Autodesk Inventor part; units mm, degrees
ref_plane "XZ Plane" through (0, 0, 0) normal (0, 1, 0) x (-1, 0, 0)
ref_plane "XY Plane" through (0, 0, 0) normal (0, 0, 1) x (1, 0, 0)
sketch "Эскиз1" plane through (0, 0, 0) normal (1, 0, 0) x (0, 1, 0)
  circle A0 centre (0, 0) radius 70
  circle A1 centre (0, 0) radius 82.5
  arc A2 (80.4212, 18.894) -> (80.3103, 18.8815) centre (82.3009, 1.7165) ccw
  circle A3 centre (0, 0) radius 97.5
  line L0 (142.5, 102) -> (108, 102)
  line L1 (0, -132.6) -> (0, 165.6)
  line L2 (142.5, 102) -> (142.5, 68)
  line L3 (108, 102) -> (108, 101.5)
  line L4 (108, 101.5) -> (0, 101.5)
  line L5 (-142.5, 102) -> (-108, 102)
  line L6 (-142.5, 102) -> (-142.5, 68)
  line L7 (-108, 102) -> (-108, 101.5)
  line L8 (-108, 101.5) -> (0, 101.5)
  arc A4 (11.7449, -38.2368) -> (27.2385, -29.2927) centre (0, 0) ccw
  arc A5 (-27.2416, -29.2898) -> (-11.749, -38.2356) centre (0, 0) ccw
  line L9 (-142.5, 68) -> (-69.8731, 68)
  line L10 (97.5, 0) -> (97.5, 68)
  line L11 (142.5, 68) -> (69.8731, 68)
  line L12 (-97.5, 0) -> (-97.5, 68)
  line L13 (117.5, 43) -> (117.5, 123)
  line L14 (-117.5, 43) -> (-117.5, 123)
  line L15 (133.5, 68) -> (117.5, 68)
  line L16 (117.5, 68) -> (117.5, 69)
  line L17 (117.5, 69) -> (133.5, 69)
  line L18 (133.5, 69) -> (133.5, 68)
  line L19 (128.5, 69) -> (117.5, 69)
  line L20 (117.5, 69) -> (117.5, 85)
  line L21 (128.5, 102) -> (128.5, 69)
  line L22 (133.5, 102) -> (117.5, 102)
  line L23 (117.5, 69) -> (101.5, 69)
  line L24 (101.5, 69) -> (101.5, 68)
  line L25 (106.5, 101.5) -> (106.5, 69)
  line L26 (-108, 102) -> (-108, 101.5)
  line L27 (-133.5, 68) -> (-117.5, 68)
  line L28 (-117.5, 68) -> (-117.5, 69)
  line L29 (-117.5, 69) -> (-133.5, 69)
  line L30 (-133.5, 69) -> (-133.5, 68)
  line L31 (-128.5, 69) -> (-117.5, 69)
  line L32 (-117.5, 69) -> (-117.5, 85)
  line L33 (-128.5, 102) -> (-128.5, 69)
  line L34 (-133.5, 102) -> (-117.5, 102)
  line L35 (-101.5, 69) -> (-101.5, 68)
  line L36 (-117.5, 69) -> (-101.5, 69)
  line L37 (-106.5, 101.5) -> (-106.5, 69)
  line L38 (117.5, 68) -> (117.5, 102)
  line L39 (-117.5, 68) -> (-117.5, 102)
  line L40 (0, 0) -> (69.6414, -69.6414)
  circle A6 centre (58.3363, -58.3363) radius 6.5
  circle A7 centre (58.3363, 58.3363) radius 6.5
  circle A8 centre (-58.3363, 58.3363) radius 6.5
  circle A9 centre (-58.3363, -58.3363) radius 6.5
  arc A10 (69.8731, 68) -> (-69.8731, 68) centre (0, 0) ccw
  line L41 (97.5, 68) -> (69.8731, 68)
  line L42 (-69.8731, 68) -> (-97.5, 68)
  line L43 (128.5, 69) -> (128.5, 102)
  line L44 (89, 68) -> (89, 101.5)
  arc A11 (83.0142, 68) -> (79.5188, 56.4182) centre (116.097, 51.6972) ccw
  arc A12 (79.5188, 56.4182) -> (62.6803, 74.6822) centre (0, 0) ccw
  line L45 (83.0142, 68) -> (83.0142, 84.568)
  line L46 (83.0142, 84.568) -> (89, 84.568)
  arc A13 (79.5188, 56.4182) -> (62.6803, 74.6822) centre (0, 0) ccw
  line L47 (-101.5, 69) -> (-101.5, 68)
  line L48 (-97.5, 68) -> (-69.8731, 68)
  arc A14 (-79.5188, 56.4182) -> (-83.0142, 68) centre (-116.097, 51.6972) ccw
  arc A15 (-62.6803, 74.6822) -> (-79.5188, 56.4182) centre (0, 0) ccw
  line L49 (-83.0142, 68) -> (-83.0142, 84.568)
  line L50 (-83.0142, 84.568) -> (-89, 84.568)
  arc A16 (-62.6803, 74.6822) -> (-79.5188, 56.4182) centre (0, 0) ccw
  line L51 (0, 97.5) -> (0, 101.5)
  line L52 (0, 101.5) -> (89, 101.5)
  line L53 (89, 101.5) -> (89, 84.568)
  arc A17 (62.6803, 74.6822) -> (0, 97.5) centre (0, 0) ccw
  arc A18 (89, 84.568) -> (47.9908, 67.1054) centre (89, 27.6838) ccw
  arc A19 (47.9908, 67.1054) -> (0, 82.5) centre (0, 0) ccw
  line L54 (79.5188, 56.4182) -> (60.3628, 70.1005)
  line L55 (60.3628, 70.1005) -> (47.9908, 67.1054)
  arc A20 (-47.9908, 67.1054) -> (-89, 84.568) centre (-89, 27.6838) ccw
  line L56 (-79.5188, 56.4182) -> (-59.1498, 66.8423)
  line L57 (-59.1498, 66.8423) -> (-47.9908, 67.1054)
  line L58 (0, 101.5) -> (-89, 101.5)
  line L59 (-89, 101.5) -> (-89, 84.568)
  arc A21 (-47.9908, 67.1054) -> (-89, 84.568) centre (-89, 27.6838) ccw
  arc A22 (0, 82.5) -> (-47.9908, 67.1054) centre (0, 0) ccw
  arc A23 (47.9908, 67.1054) -> (-47.9908, 67.1054) centre (0, 0) ccw
  point P0 (80.4117, 18.4447)
  point P1 (0, -97.5)
  point P2 (128.5, 85)
  point P3 (106.5, 85)
  point P4 (-128.5, 85)
  point P5 (-106.5, 85)
  point P6 (-89, 68)
  dimension "d0" = 140
  dimension "d4" = 165
  dimension "d19" = 195
  dimension "d20" = 199.5
  dimension "d22" = 285
  dimension "d23" = 216
  dimension "d24" = 0.5
  dimension "d46" = 34
  dimension "d64" = 235
  dimension "d65" = 16
  dimension "d66" = 11
  dimension "d67" = 1
  dimension "d70" = 45
  dimension "d71" = 13
  dimension "d74" = 360
  dimension "d84" = 12.5
extrude "Выдавливание1" add sketch "Эскиз1" along normal blind 34 and the other way blind 34 contours A0 L1 A1 A7 A6 L40 | A0 L1 A1 A9 A8 | L40 A6 A1 L1 A0 | A6 A1 L40 | L40 A1 A6 | A1 A9 | A1 A7 | A8 A1 picked at (57.6773, -55.9908) picked at (55.9908, -57.6773) picked at (-56.6588, -56.9353) picked at (56.9815, 56.6214) picked at (-56.6588, 56.9353)
extrude "Выдавливание2" add sketch "Эскиз1" along normal blind 34 and the other way blind 34 contours A0 L40 L1 | A0 L1 A1 A7 A6 L40 | L1 A0 | A0 L1 A1 A9 A8 | L40 A6 A1 L1 A0 | A0 L1 L40 | A6 A1 L40 | L40 A1 A6 | A1 A9 | A1 A7 | A8 A1 picked at (57.6773, -55.9908) picked at (55.9908, -57.6773) picked at (-56.6588, -56.9353) picked at (56.9815, 56.6214) picked at (-56.6588, 56.9353)
pattern_circular "Круговой массив1" count 6 over 360 about axis through (0, 0, 0) along (1, 0, 0) of "Выдавливание2"
extrude "Выдавливание3" add sketch "Эскиз1" along normal blind 33 and the other way blind 33 contours A0 L40 L1 | A0 L1 A1 A7 A6 L40 | L1 A0 | A0 L1 A1 A9 A8 | L40 A6 A1 L1 A0 | A0 L1 L40 | L1 A3 A18 A1 | A1 A20 A3 L1 | A6 A1 L40 | L40 A1 A6 | L1 A3 L56 L57 A1 A8 A9 | A1 A6 L40 A3 L1 | L55 L54 A3 L40 A6 A1 A7 | A18 A3 L54 L55 | L57 L56 A3 A20 | L40 A6 A1 | A1 A6 L40 | A9 A1 | A1 A9 | A7 A1 | A1 A7 | A8 A1 | A1 A8 | A11 L11 L10 A3 | A3 L11 A11
extrude "Выдавливание4" add sketch "Эскиз1" along normal blind 33 and the other way blind 33 contours L12 L9 A14 A3 | A14 L9 A3
extrude "Выдавливание7" add sketch "Эскиз1" along normal blind 33 and the other way blind 33 contours A0 L40 L1 | A0 L1 A1 A7 A6 L40 | L1 A0 | A0 L1 A1 A9 A8 | L40 A6 A1 L1 A0 | A0 L1 L40 | L1 A3 A18 A1 | A1 A20 A3 L1 | L1 A3 L56 L57 A1 A8 A9 | A1 A6 L40 A3 L1 | L55 L54 A3 L40 A6 A1 A7 | A18 A3 L54 L55 | L57 L56 A3 A20 | L1 L4 L44 L46 L45 A18 A3 | A3 A20 L49 L50 L59 L8 L1 | A18 L45 L11 A3 | A3 L9 L49 A20 | A18 L44 L11 L45 | L45 L46 A18 | A20 L50 L49 | L49 L9 L35 L36 L37 L8 L59 A20 | L4 L25 L23 L24 L11 L44 | L37 L36 L14 L5 L7 L8 | L9 L14 L36 L35 | L23 L13 L11 L24 | L9 L30 L29 L14 | L17 L18 L11 L13 | L29 L33 L5 L14 | L9 L6 L5 L33 L29 L30 | L21 L0 L2 L11 L18 L17
extrude "Выдавливание8" add sketch "Эскиз1" along normal blind 33 and the other way blind 33 contours L4 L3 L0 L13 L23 L25 | L17 L18 L11 L13 | L13 L0 L21 L17 | L21 L0 L2 L11 L18 L17
revolve "Вращение2" cut sketch "Эскиз1" angle 360 about axis through (0, -117.5, 43) along (0, 0, 1) contours L9 L30 L29 L14 | L29 L33 L5 L14
extrude "Выдавливание9" add sketch "Эскиз1" along normal blind 33 and the other way blind 33 contours A18 L44 L11 L45 | L45 L46 A18 | L4 L25 L23 L24 L11 L44 | L23 L13 L11 L24 | L17 L18 L11 L13
extrude "Выдавливание11" [suppressed]
revolve "Вращение1" cut sketch "Эскиз1" angle 360 about axis through (0, 117.5, 43) along (0, 0, 1) contours L17 L18 L11 L13 | L13 L0 L21 L17
extrude "Выдавливание12" cut sketch "Эскиз1" along normal blind 21 and the other way blind 21 contours L1 A3 A18 A1 | A1 A20 A3 L1 | L1 L4 L44 L46 L45 A18 A3 | A3 A20 L49 L50 L59 L8 L1 | L45 L46 A18 | A20 L50 L49
extrude "Выдавливание13" cut sketch "Эскиз1" along normal through all both and the other way through all contours A6 A1 L40 | L40 A1 A6 | L40 A6 A1 | A1 A6 L40 | A9 A1 | A1 A9 | A7 A1 | A1 A7 | A8 A1 | A1 A8
extrude "Выдавливание14" cut sketch "Эскиз1" along normal through all both and the other way through all contours A0 L40 L1 | L1 A0 | A0 L1 L40
sketch "Эскиз3" plane through (34, 0, 0) normal (1, 0, 0) x (0, 0, -1)
  line L0 (-68, 97.5) -> (-68, 142.5)
  line L1 (-68, 97.5) -> (-68, 86.5)
  line L2 (-68, 86.5) -> (-85, 67.5)
  line L3 (-85, 67.5) -> (-101.5, 67.5)
  line L4 (-101.5, 89) -> (-101.5, -89)
  line L5 (-101.5, 67.5) -> (-101.5, 0)
  arc A0 (0, 97.5) -> (0, 97.5) centre (0, 0) ccw
  line L6 (-68, 97.5) -> (-52.0783, 73.402)
  line L7 (137.4, 0) -> (-141.9, 0)
  line L8 (-68, -97.5) -> (-64, -83.0142)
  line L9 (-68, -97.5) -> (-68, -86.5)
  line L10 (-68, -86.5) -> (-85, -67.5)
  line L11 (-85, -67.5) -> (-101.5, -67.5)
  line L12 (-101.5, -67.5) -> (-101.5, 0)
  line L13 (-68, -97.5) -> (-52.0783, -73.402)
  arc A1 (-64, 83.0142) -> (-52.0783, 73.402) centre (-35.394, 106.294) ccw
  arc A2 (-52.0783, -73.402) -> (-64, -83.0142) centre (-35.394, -106.294) ccw
  arc A3 (-52.0783, 73.402) -> (-52.0783, -73.402) centre (0, 0) ccw
  point P0 (-68, 142.5)
extrude "Выдавливание15" [suppressed]
extrude "Выдавливание16" [suppressed]
sketch "Эскиз4" plane through (-34, 0, 0) normal (-1, 0, 0) x (0, -1, 0)
  circle A0 centre (-58.3363, -58.3363) radius 6.5
  arc A1 (-66.7759, -48.4482) -> (-58.3363, -58.3363) centre (0, 0) ccw
  arc A2 (-66.7759, -48.4482) -> (-48.4482, -66.7759) centre (-58.3363, -58.3363) ccw
  arc A3 (-58.3363, -58.3363) -> (-48.4482, -66.7759) centre (0, 0) ccw
  arc A4 (-62.7479, -53.5626) -> (-53.5626, -62.7479) centre (-58.3363, -58.3363) ccw
  arc A5 (-53.5626, -62.7479) -> (-48.4482, -66.7759) centre (0, 0) ccw
  arc A6 (-66.7759, -48.4482) -> (-62.7479, -53.5626) centre (0, 0) ccw
  arc A7 (48.4482, -66.7759) -> (58.3363, -58.3363) centre (0, 0) ccw
  arc A8 (48.4482, -66.7759) -> (66.7759, -48.4482) centre (58.3363, -58.3363) ccw
  arc A9 (58.3363, -58.3363) -> (66.7759, -48.4482) centre (0, 0) ccw
  arc A10 (53.5626, -62.7479) -> (62.7479, -53.5626) centre (58.3363, -58.3363) ccw
  arc A11 (62.7479, -53.5626) -> (66.7759, -48.4482) centre (0, 0) ccw
  arc A12 (48.4482, -66.7759) -> (53.5626, -62.7479) centre (0, 0) ccw
  arc A13 (66.7759, 48.4482) -> (58.3363, 58.3363) centre (0, 0) ccw
  arc A14 (66.7759, 48.4482) -> (48.4482, 66.7759) centre (58.3363, 58.3363) ccw
  arc A15 (58.3363, 58.3363) -> (48.4482, 66.7759) centre (0, 0) ccw
  arc A16 (62.7479, 53.5626) -> (53.5626, 62.7479) centre (58.3363, 58.3363) ccw
  arc A17 (53.5626, 62.7479) -> (48.4482, 66.7759) centre (0, 0) ccw
  arc A18 (66.7759, 48.4482) -> (62.7479, 53.5626) centre (0, 0) ccw
  arc A19 (-48.4482, 66.7759) -> (-58.3363, 58.3363) centre (0, 0) ccw
  arc A20 (-48.4482, 66.7759) -> (-66.7759, 48.4482) centre (-58.3363, 58.3363) ccw
  arc A21 (-58.3363, 58.3363) -> (-66.7759, 48.4482) centre (0, 0) ccw
  arc A22 (-53.5626, 62.7479) -> (-62.7479, 53.5626) centre (-58.3363, 58.3363) ccw
  arc A23 (-62.7479, 53.5626) -> (-66.7759, 48.4482) centre (0, 0) ccw
  arc A24 (-48.4482, 66.7759) -> (-53.5626, 62.7479) centre (0, 0) ccw
  arc A25 (-66.7759, -48.4482) -> (-48.4482, -66.7759) centre (0, 0) ccw
  arc A26 (-66.7759, -48.4482) -> (-48.4482, -66.7759) centre (0, 0) ccw
  arc A27 (-66.7759, -48.4482) -> (-48.4482, -66.7759) centre (0, 0) ccw
  arc A28 (-66.7759, -48.4482) -> (-48.4482, -66.7759) centre (-58.3363, -58.3363) ccw
  dimension "d112" = 360
  dimension "d116" = 360
  dimension "d118" = 13
equation "\"d0\" = D"
equation "\"d4\" = D1"
equation "\"d19\" = -2 * H1 + 2 * H_"
equation "\"d20\" = H_"
equation "\"d22\" = L"
equation "\"d23\" = t"
equation "\"d46\" = h_"
equation "\"d64\" = L2"
equation "\"d65\" = 0.5 * d3"
equation "\"d66\" = 0.5 * d1"
equation "\"d71\" = d"
equation "\"d25\" = 0.5 * B"
equation "\"d26\" = 0.5 * B"
equation "\"d34\" = 0.5 * B"
equation "\"d35\" = 0.5 * B"
equation "\"d76\" = 0.5 * B1"
equation "\"d77\" = 0.5 * B1"
equation "\"d80\" = 0.5 * B1"
equation "\"d81\" = 0.5 * B1"
equation "\"d85\" = 0.5 * B1"
equation "\"d86\" = 0.5 * B1"
equation "\"d94\" = 0.5 * B1"
equation "\"d95\" = 0.5 * B"
equation "\"D\" = 140"
equation "\"D1\" = 165"
equation "\"d\" = 13"
equation "\"del\" = 0.12"
equation "\"d1\" = 22"
equation "\"L2\" = 235"
equation "\"B\" = 68"
equation "\"B1\" = 66"
equation "\"L\" = 285"
equation "\"L1\" = 195"
equation "\"t\" = 216"
equation "\"H_\" = 199.5"
equation "\"H1\" = 102"
equation "\"h_\" = 34"
equation "\"d3\" = 32"
properties part number "корпус подшипника1"
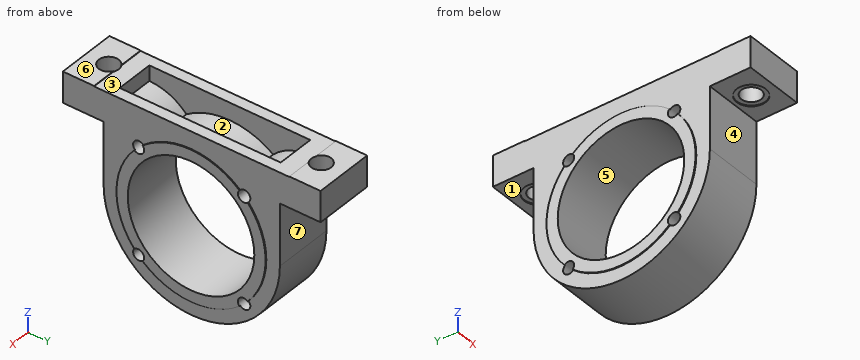
Verification items for the finished model (mm, model axes). Face numbers are marked on the shaded views. A direction names the side the tool comes from. Round coordinates to 2 decimals unless told otherwise and drop trailing zeros. Write each loop counter-clockwise with the first axis right and the second up, starting at its lowest first coordinate (ties: lowest second). Pieces come first, ordered by that corner, then holes. Notation, with made-up numbers: (8, 36) -> (53, 36) arc R16 cw to (53, 45) -> close; hole circle Ø3 at (10.25, 5). An arc over 180 degrees is marked (long way). Write each question's results on one line, items separated by ' | '.
Q1. Sectioned sample at A-A, the plane y = -117.5. Record the boundary of the cut face in (x, z), and give its area (3 significant figures).
Derived:
outline: (-33, 68) -> (-16, 68) -> (-16, 69) -> (-11, 69) -> (-11, 102) -> (-33, 102) -> close; (11, 69) -> (16, 69) -> (16, 68) -> (33, 68) -> (33, 102) -> (11, 102) -> close | area: 1,490 mm²
Q2. Go/stop test with flat-tipped pins: pin 1 Ø2 at (x, z) = (-17, -34) entering from +Y; pin 2 Ø1 at (x, z) = (13, -64) entering from +Y; pin 3 Ø4 at (x, z) = (-6, -45.5) entering from +Y. Record where each tip stops, or that it passes through.
Derived:
pin 1: stops at y = 91.75 | pin 2: stops at y = 73.99 | pin 3: stops at y = 87.26
Q3. Draft check along Z on the marked faces 5, 6 and 7. Enter one of: released by +Z, released by -Z, zero draft, split by the parting line, or undercut.
Derived:
face 5: undercut | face 6: released by +Z | face 7: zero draft
Q4. Sectioned sample at D-D, the plane x = 0. Give the number of separate pieces and of enclosed holes in the cut face, and give its area (3 significant figures).
Derived:
separate pieces: 3 | enclosed holes: 5 | area: 16,200 mm²
Q5. Sectioned sample at B-B, the plane z = 48. Record the boundary of the cut face in (x, y).
Derived:
outline: (-34, -67.1) -> (-33, -67.1) -> (-33, -97.5) -> (33, -97.5) -> (33, -67.1) -> (34, -67.1) -> (34, -50.95) -> (-34, -50.95) -> close; (-34, 50.95) -> (34, 50.95) -> (34, 67.1) -> (33, 67.1) -> (33, 97.5) -> (-33, 97.5) -> (-33, 67.1) -> (-34, 67.1) -> close
Q6. Sectioned sample at C-C, the plane x = 26. Record the boundary of the cut face in (y, z), and give its area (3 significant figures).
Derived:
outline: (-142.5, 68) -> (-97.5, 68) -> (-97.5, 0) arc R97.5 ccw to (97.5, 0) -> (97.5, 68) -> (142.5, 68) -> (142.5, 102) -> (108, 102) -> (108, 101.5) -> (-108, 101.5) -> (-108, 102) -> (-142.5, 102) -> close; hole circle Ø140 at (0, 0); hole circle Ø13 at (-58.34, -58.34); hole circle Ø13 at (-58.34, 58.34); hole circle Ø13 at (58.34, -58.34); hole circle Ø13 at (58.34, 58.34) | area: 21,800 mm²
Q7. Thickness scan on probe 1 along Y at (x, z) = (0, 89); probe 2 along Z at (x, y) = (13.5, 0.5); probe 3 along Z at (x, y) = (14, -62). Record the ranges inside material, lowest first.
Derived:
probe 1: y = -142.5 to -128.5, -106.5 to -89, 89 to 106.5, 128.5 to 142.5 | probe 2: z = -97.5 to -70, 70 to 82.5 | probe 3: z = -75.25 to -63.71, -52.97 to -32.5, 32.5 to 52.97, 63.71 to 77.75
Q8. Access from +Z, -Z, +X, -X, +Y, -Y to the whole of each face (thin tool, end or side, straight path). Record for the marked faces 1, 2, 3 and 4.
Derived:
face 1: -Z, +X, -X, +Y | face 2: +Z | face 3: +Z, +X, -X | face 4: -Z, +X, -X, -Y
